from build123d import *

# Parameters (mm, degrees)
SKETCH1_W           = 70.104
SKETCH1_H           = 31.75
BOSS_EXTRUDE1_DEPTH = 3.175
SKETCH2_W           = 3.2258
SKETCH2_H           = 6.35
TABS_DEPTH          = 3.175


with BuildPart() as part:
    # Sketch1 → Boss-Extrude1 (new body)
    with BuildSketch(Plane(origin=(0, 0, 0), x_dir=(1, 0, 0), z_dir=(0, 1, 0))):
        Rectangle(SKETCH1_W, SKETCH1_H)
    extrude(amount=BOSS_EXTRUDE1_DEPTH)

    # Sketch2 → tabs (add)
    with BuildSketch(Plane(origin=(0, 3.175, 0), x_dir=(1, 0, 0), z_dir=(0, 1, 0))):
        with Locations((-36.6649, 9.525)):
            Rectangle(SKETCH2_W, SKETCH2_H)
        with Locations((-36.6649, -9.525)):
            Rectangle(SKETCH2_W, SKETCH2_H)
    tabs = extrude(amount=-TABS_DEPTH)

    # Mirror1: tabs across plane
    add(tabs.mirror(Plane(origin=(0, 0, 0), x_dir=(0, 0, 1), z_dir=(1, 0, 0))))


solid = part.part
Design review of the part built by this model. Coordinates are the model's own, in mm. A direction names the side the tool comes from. Give positions to 0.01 mm unless a question says otherwise; leave off trailing zeros. Loops run counter-clockwise (first coordinate to the right, second up) from the corner with the lowest first, then second, coordinate; pieces in that order, holes last. Notation, with made-up numbers: M 29,10 L 42,10 A35 cw 42,46 Z; hole C 28.5,0 d5. An arc over 180 degrees is marked long. One line per question, with ' | ' between items. Start each with the question number.
1. For faces 1 (the face through (-37, 2, -6.35)), 2 (the face through (-37, 2, 12.7)), 3 (the face through (-35.052, 2, -14)), list the 3-axis set-ups (+Z, -Z, +X, -X, +Y, -Y) from which the entire face can be reached by the end or side of a thin tool; tool diameter is ignored.
2. To check wall thickness, follow L1, parallel to X at y = 1.6, z = -4. State the ranges of the line that lie inside material, in increasing order.
3. Add section B-B (z = 1). Write out the cut boundary in (x, y) (3 decimals), plus the area to 3 significant figures.
4. Insertion check: P1, Ø1, axis at x = -36.5, y = 1, coming from the +Z side; P2, Ø1.6, axis at y = 2, z = 14.5, coming from the -X side; P3, Ø1.6, axis at x = -36, y = 1, coming from the -Z side. Each pin has a flat end and moves straight along its axis. Give the tip position at first contact, or say it passes through.
5. Add section A-A (y = 1.6). Write out the cut boundary in (x, z) (3 decimals).
Worked out:
1) face 1: -X, +Y, -Y | face 2: +Z, -X, +Y, -Y | face 3: -Z, -X, +Y, -Y
2) L1: x = -35.05 to 35.05
3) outline: M -35.052,0 L 35.052,0 L 35.052,3.175 L -35.052,3.175 Z | area: 223 mm²
4) P1: stops at z = 12.7 | P2: stops at x = -35.05 | P3: stops at z = -12.7
5) outline: M -38.278,-12.7 L -35.052,-12.7 L -35.052,-15.875 L 35.052,-15.875 L 35.052,-12.7 L 38.278,-12.7 L 38.278,-6.35 L 35.052,-6.35 L 35.052,6.35 L 38.278,6.35 L 38.278,12.7 L 35.052,12.7 L 35.052,15.875 L -35.052,15.875 L -35.052,12.7 L -38.278,12.7 L -38.278,6.35 L -35.052,6.35 L -35.052,-6.35 L -38.278,-6.35 Z
